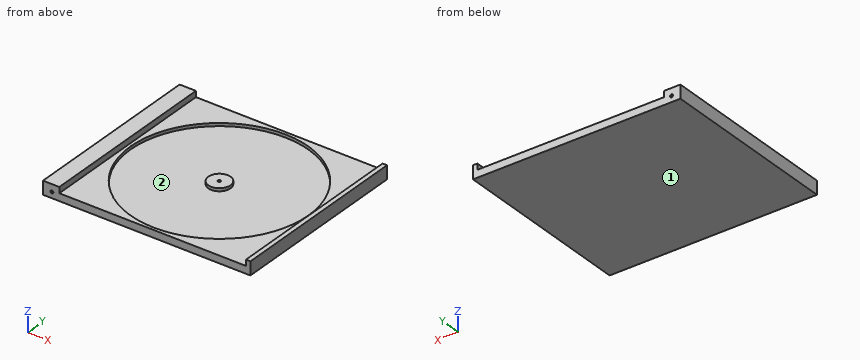
from build123d import *

# Parameters (mm, degrees)
F0_W      = 140
F0_H      = 124
F1_DEPTH  = 5
F2_W      = 11
F2_H      = 124
F2_W_2    = 3
F3_DEPTH  = 4
F5_DEPTH  = 2
F6_DEPTH  = 2
F7_R      = 1
F8_DEPTH  = 1
F9_R      = 1
F10_DEPTH = 1


with BuildPart() as f1:
    # F0 (on Top) → F1 (new body)
    with BuildSketch(Plane.XY):
        Rectangle(F0_W, F0_H)
    extrude(amount=-F1_DEPTH)

    # F2 (on face) → F3 (join)
    with BuildSketch(Plane.XY):
        with Locations((-64.5, 0)):
            Rectangle(F2_W, F2_H)
        with Locations((68.5, 0)):
            Rectangle(F2_W_2, F2_H)
    extrude(amount=F3_DEPTH)

    # F4 (on face) → F5 (cut)
    with BuildSketch(Plane.XY):
        with BuildLine():
            ThreePointArc((3, 7.5), (8.3033008589, 5.3033008589), (10.5, 0))
            Line((10.5, 0), (63, 0))
            ThreePointArc((63, 0), (45.4264068712, 42.4264068712), (3, 60))
            Line((3, 60), (3, 7.5))
        make_face()
        with BuildLine():
            Line((63, 0), (10.5, 0))
            ThreePointArc((10.5, 0), (8.3033008589, -5.3033008589), (3, -7.5))
            Line((3, -7.5), (3, -60))
            ThreePointArc((3, -60), (45.4264068712, -42.4264068712), (63, 0))
        make_face()
        with BuildLine():
            ThreePointArc((-4.5, 0), (-2.3033008589, 5.3033008589), (3, 7.5))
            Line((3, 7.5), (3, 60))
            ThreePointArc((3, 60), (-39.4264068712, 42.4264068712), (-57, 0))
            Line((-57, 0), (-4.5, 0))
        make_face()
        with BuildLine():
            Line((3, -60), (3, -7.5))
            ThreePointArc((3, -7.5), (-2.3033008589, -5.3033008589), (-4.5, 0))
            Line((-4.5, 0), (-57, 0))
            ThreePointArc((-57, 0), (-39.4264068712, -42.4264068712), (3, -60))
        make_face()
    extrude(amount=-F5_DEPTH, mode=Mode.SUBTRACT)

    # F4 (on face) → F6 (cut)
    with BuildSketch(Plane.XY):
        with BuildLine():
            ThreePointArc((3, -1), (3.7071067812, -0.7071067812), (4, 0))
            Line((4, 0), (3, 0))
            Line((3, 0), (3, -1))
        make_face()
        with BuildLine():
            Line((3, -1), (3, 0))
            Line((3, 0), (2, 0))
            ThreePointArc((2, 0), (2.2928932188, -0.7071067812), (3, -1))
        make_face()
        with BuildLine():
            Line((2, 0), (3, 0))
            Line((3, 0), (3, 1))
            ThreePointArc((3, 1), (2.2928932188, 0.7071067812), (2, 0))
        make_face()
        with BuildLine():
            Line((3, 0), (4, 0))
            ThreePointArc((4, 0), (3.7071067812, 0.7071067812), (3, 1))
            Line((3, 1), (3, 0))
        make_face()
    extrude(amount=-F6_DEPTH, mode=Mode.SUBTRACT)

    # F7 (on face) → F8 (cut)
    with BuildSketch(Plane(origin=(0, 62, 0), x_dir=(-1, 0, 0), z_dir=(0, 1, 0))):
        with Locations((64, -1)):
            Circle(F7_R)
    extrude(amount=-F8_DEPTH, mode=Mode.SUBTRACT)

    # F9 (on face) → F10 (cut)
    with BuildSketch(Plane.XZ.offset(62)):
        with Locations((-64, -1)):
            Circle(F9_R)
    extrude(amount=-F10_DEPTH, mode=Mode.SUBTRACT)


solid = f1.part
Read the model definition and answer for the solid it produces. Units are mm, in the model's axes. Face numbers are marked on the shaded views. Coordinates: 2 decimals unless noted, no trailing zeros. Write each loop counter-clockwise with the first axis right and the second up, starting at its lowest first coordinate (ties: lowest second). Pieces come first, ordered by that corner, then holes. Notation, with made-up numbers: (70.5, -23) - (93.5, -23) arc R11 ccw to (93.5, -3) - close; hole circle Ø5 at (-25, -24.5). An arc over 180 degrees is marked (long way). One line per question, with ' | ' between items.
Q1. Find section D-D, the plane y = 5. Write down the section's boundary in (x, z).
Result set:
outline: (-70, -5) - (70, -5) - (70, 4) - (67, 4) - (67, 0) - (62.79, 0) - (62.79, -2) - (8.59, -2) - (8.59, 0) - (-2.59, 0) - (-2.59, -2) - (-56.79, -2) - (-56.79, 0) - (-59, 0) - (-59, 4) - (-70, 4) - close
Q2. Find section C-C, the plane x = -53.5. Write down the section's boundary in (y, z), plus the area to 3 significant figures.
Result set:
outline: (-62, -5) - (62, -5) - (62, 0) - (20.19, 0) - (20.19, -2) - (-20.19, -2) - (-20.19, 0) - (-62, 0) - close | area: 539 mm^2
Q3. Consider L1, parallel to Y at x = 3, z = -0.7; L2, parallel to Z at x = -64, y = -61.25; L3, parallel to X at y = 23, z = 2.25. Determine where each line is inside the solid, lowest interval first. Write a range as [from, to].
Result set:
L1: [-62, -60], [-7.5, -1], [1, 7.5], [60, 62] | L2: [-5, -2], [0, 4] | L3: [-70, -59], [67, 70]
Q4. Find section B-B, the plane y = -40. Write down the section's boundary in (x, z), plus the area to 3 significant figures.
Result set:
outline: (-70, -5) - (70, -5) - (70, 4) - (67, 4) - (67, 0) - (47.72, 0) - (47.72, -2) - (-41.72, -2) - (-41.72, 0) - (-59, 0) - (-59, 4) - (-70, 4) - close | area: 577 mm^2
Q5. Determine the mould class of the marked faces 1 and 2 for opening direction X: +X half, -X half, draft (parallel to the pull), parting line (faces both ways), or undercut.
Result set:
face 1: draft | face 2: undercut
Q6. Find section A-A, the plane z = 1.5. Write down the section's boundary in (x, y), plus the area to 3 significant figures.
Result set:
outline: (-70, -62) - (-59, -62) - (-59, 62) - (-70, 62) - close; (67, -62) - (70, -62) - (70, 62) - (67, 62) - close | area: 1,740 mm^2
Q7. Each of these flat-tipped pins is pushed along its axis until it touches: P1, Ø4.5, axis at x = 5, y = -1.5, coming from the +Z side; P2, Ø1.8, axis at x = -64, z = -1, coming from the +Y side; P3, Ø1, axis at x = 10, y = 26, coming from the +Z side; P4, Ø2.5, axis at x = -64, z = -1, coming from the -Y side. Where does it stop, or does it pass through?
Result set:
P1: z = 0 | P2: y = 61 | P3: z = -2 | P4: y = -62
